Here's the drawing with two shaded views (mm, measured from the low corner). I have some questions. Coordinates: 2 decimals unless noted, no trailing zeros. Write each loop counter-clockwise with the first axis right and the second up, starting at its lowest first coordinate (ties: lowest second). Pieces come first, ordered by that corner, then holes.
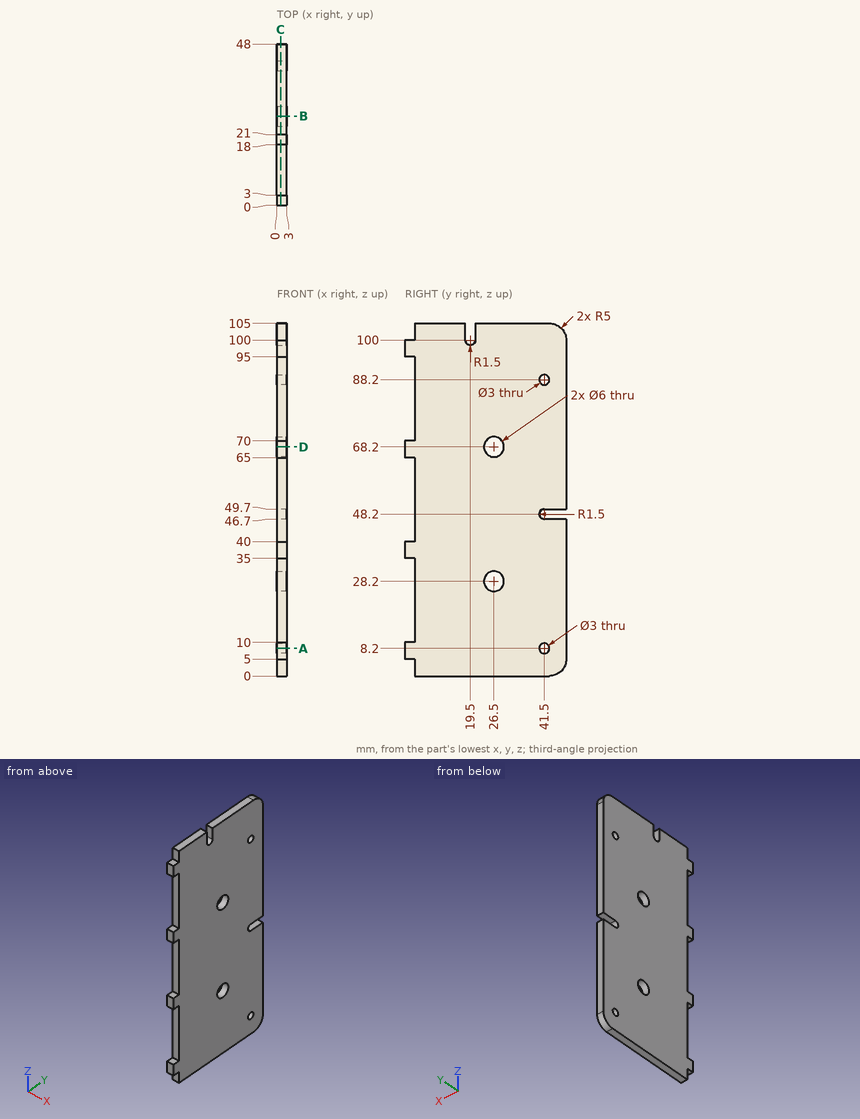
Item 1: I want a section at C-C, the plane x = 1.15. Count the separate pieces of the cut face and the enclosed holes in it, then the cut area to 3 significant figures.
Item 2: I want a section at B-B, the plane y = 26.5. List the corners of the cut face in (x, z) for me.
Item 3: If I drill on line 1 along Y through (x, z) = (0.8, 68.2); line 2 along Z through (x, y) = (0.35, 28); line 3 along Y through (x, z) = (1.5, 58.5), over which ranges is the centre line in solid material (lowest first)?
Item 4: I want a section at A-A, the plane z = 8.2. List the corners of the cut face in (x, y) for me.
Item 5: Will these pins go through, and if not, where does the flat tip stop? pin 1 Ø1.5 at (x, y) = (2, 2) entering from +Z; pin 2 Ø1.5 at (x, y) = (1, 2) entering from -Z; pin 3 Ø1.5 at (x, z) = (1, 24) entering from -Y.
Item 6: I want a section at D-D, the plane z = 68.2. List the corners of the cut face in (x, y) for me, then the cut area to 3 significant figures.
Taken from the geometry:
1. separate pieces: 1
1. enclosed holes: 4
1. area: 4,660 mm2
2. outline: (0, 0) - (3, 0) - (3, 25.2) - (0, 25.2) - close; (0, 31.2) - (3, 31.2) - (3, 65.2) - (0, 65.2) - close; (0, 71.2) - (3, 71.2) - (3, 105) - (0, 105) - close
3. line 1: y = 0 to 23.5, 29.5 to 48
3. line 2: z = 0 to 25.6, 30.8 to 65.6, 70.8 to 105
3. line 3: y = 3 to 48
4. outline: (0, 0) - (3, 0) - (3, 40) - (0, 40) - close; (0, 43) - (3, 43) - (3, 48) - (0, 48) - close
5. pin 1: stops at z = 100
5. pin 2: stops at z = 5
5. pin 3: stops at y = 3
6. outline: (0, 0) - (3, 0) - (3, 23.5) - (0, 23.5) - close; (0, 29.5) - (3, 29.5) - (3, 48) - (0, 48) - close
6. area: 126 mm2
